The model under review builds one solid part; all positions refer to its coordinate system, in mm. A direction names the side the tool comes from. Coordinates: 2 decimals unless noted, no trailing zeros. Order: outer loops, then holes, each group sorted by start corner. A loop starts at its lowest first (then second) coordinate and runs counter-clockwise, first axis right, second up. Notation, with made-up numbers: (55.25, 45.25) -> (112.25, 45.25) arc R26 cw to (112.25, 62.25) -> close; hole circle Ø8 at (70.5, -32.75). An arc over 180 degrees is marked (long way). Use one line per item in the form item = value.
from build123d import *

# Parameters (mm, degrees)
SKETCH1_R           = 4.5
SKETCH1_R_2         = 0.375
BOSS_EXTRUDE1_DEPTH = 0.5
SKETCH2_R           = 3
SKETCH2_R_2         = 0.35
BOSS_EXTRUDE2_DEPTH = 3
FILLET1_R           = 0.5
FILLET2_R           = 0.2


with BuildPart() as part:
    # Sketch1 → Boss-Extrude1 (new body)
    with BuildSketch(Plane(origin=(0, 0, 0), x_dir=(1, 0, 0), z_dir=(0, 1, 0))):
        with Locations(Location((0, 0, 0), (0, 0, 270))):
            Circle(SKETCH1_R)
        with Locations(Location((0, 0, 0), (0, 0, 270))):
            Circle(SKETCH1_R_2, mode=Mode.SUBTRACT)
    extrude(amount=BOSS_EXTRUDE1_DEPTH)

    # Sketch2 → Boss-Extrude2 (add)
    with BuildSketch(Plane(origin=(0, 0.5, 0), x_dir=(1, 0, 0), z_dir=(0, 1, 0))):
        with Locations(Location((0, 0, 0), (0, 0, 270))):
            Circle(SKETCH2_R)
        with Locations(Location((0, 0, 0), (0, 0, 270))):
            Circle(SKETCH2_R_2, mode=Mode.SUBTRACT)
    extrude(amount=BOSS_EXTRUDE2_DEPTH)

    # Fillet1
    fillet1_edges = [part.edges().sort_by_distance(p)[0] for p in [
        (0, 3.5, -3),
    ]]
    fillet(fillet1_edges, radius=FILLET1_R)

    # Fillet2
    fillet2_edges = [part.edges().sort_by_distance(p)[0] for p in [
        (0, 0.5, -4.5),
    ]]
    fillet(fillet2_edges, radius=FILLET2_R)


solid = part.part
Item 1: To check wall thickness, follow L1, parallel to X at y = 1.3, z = 0; L2, parallel to Y at x = 3, z = 2.75; L3, parallel to Z at x = 0.25, y = 2.85. State the ranges of each line that lie inside material, in increasing order. Write a range as from..to.
Results found:
L1 = -3..-0.35, 0.35..3
L2 = 0..0.5
L3 = -2.99..-0.24, 0.24..2.99
Item 2: We need section B-B (x = 0). Write out the cut boundary in (y, z) (3 decimals), plus the area to 3 significant figures.
Results found:
outline = (0, -4.5) -> (0.3, -4.5) arc R0.2 ccw to (0.5, -4.3) -> (0.5, -3) -> (3, -3) arc R0.5 ccw to (3.5, -2.5) -> (3.5, -0.35) -> (0.5, -0.35) -> (0.5, -0.375) -> (0, -0.375) -> close; (0, 0.375) -> (0.5, 0.375) -> (0.5, 0.35) -> (3.5, 0.35) -> (3.5, 2.5) arc R0.5 ccw to (3, 3) -> (0.5, 3) -> (0.5, 4.3) arc R0.2 ccw to (0.3, 4.5) -> (0, 4.5) -> close
area = 19.9 mm²
Item 3: We need section A-A (z = 0). Write out the cut boundary in (x, y) (3 decimals).
Results found:
outline = (-4.5, 0) -> (-0.375, 0) -> (-0.375, 0.5) -> (-0.35, 0.5) -> (-0.35, 3.5) -> (-2.5, 3.5) arc R0.5 ccw to (-3, 3) -> (-3, 0.5) -> (-4.3, 0.5) arc R0.2 ccw to (-4.5, 0.3) -> close; (0.35, 0.5) -> (0.375, 0.5) -> (0.375, 0) -> (4.5, 0) -> (4.5, 0.3) arc R0.2 ccw to (4.3, 0.5) -> (3, 0.5) -> (3, 3) arc R0.5 ccw to (2.5, 3.5) -> (0.35, 3.5) -> close
Item 4: Tool access review of faces 1 (the face through (0.9, 1.73, 2.86)), 2 (the face through (3.04, 0.15, -3.32)): name each direction out of +Z, -Z, +X, -X, +Y, -Y from which nothing blocks a thin tool from reaching the whole face with its end or side.
Results found:
face_1 = +Y
face_2 = +Y, -Y
Item 5: We need section C-C (y = 2.5). Write out the cut boundary in (x, z), plus the area to 3 significant figures.
Results found:
outline = circle Ø6 at (0, 0); hole circle Ø0.7 at (0, 0)
area = 27.9 mm²
Item 6: Clearance check with flat-ended pins moving along their axes: pin 1 (1.5 mm diameter, centred on x = 2.5, y = 2.5, fed in from -Z); pin 2 (1.5 mm diameter, centred on x = -1, y = 2, fed in from +Z). State where each tip first meets the part, or that it passes through.
Results found:
pin_1 = -2.44
pin_2 = 2.99
